Geometry: see drawing. Coordinates: mm, zero at the bounding-box minimum. A direction names the side the tool comes from. Give positions to 0.01 mm unless a question says otherwise; leave off trailing zeros. Write each loop counter-clockwise with the first axis right and the second up, starting at its lowest first coordinate (ties: lowest second). Pieces come first, ordered by that corner, then holes. Notation, with made-up numbers: (72, 10) -> (105, 10) arc R36 ccw to (105, 46) -> close; hole circle Ø1 at (50.25, 73.5). An arc over 180 degrees is marked (long way). Write item = value, one per line.
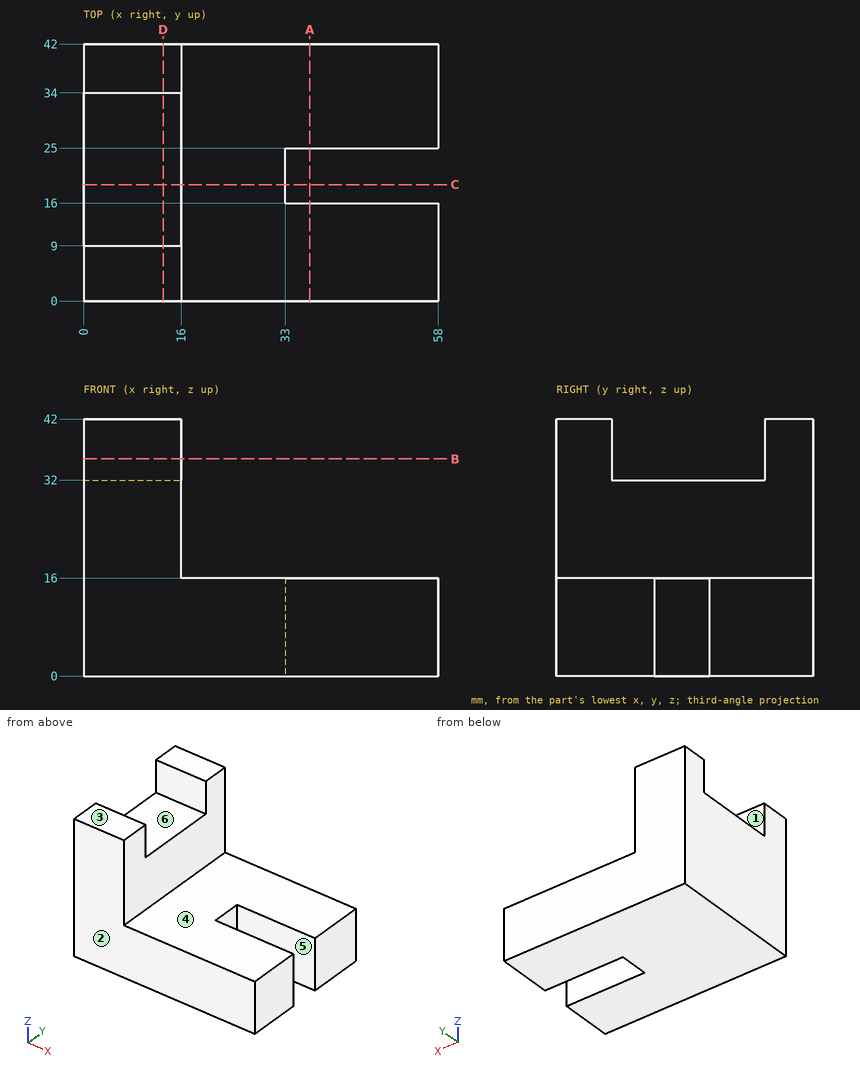
(1) Section query A-A (x = 37). Return loops of the section in (y, z), plus the area to 3 significant figures.
Values follow:
outline = (0, 0) -> (16, 0) -> (16, 16) -> (0, 16) -> close; (25, 0) -> (42, 0) -> (42, 16) -> (25, 16) -> close
area = 528 mm2
(2) Material intervals for line 1 (Y direction, x = 42.5, z = 10); line 2 (X direction, y = 24.5, z = 4); line 3 (X direction, y = 16, z = 29), sorted ascending.
Values follow:
line_1 = 0 to 16, 25 to 42
line_2 = 0 to 33
line_3 = 0 to 16
(3) Section query B-B (z = 35.5). Return loops of the section in (x, y).
Values follow:
outline = (0, 0) -> (16, 0) -> (16, 9) -> (0, 9) -> close; (0, 34) -> (16, 34) -> (16, 42) -> (0, 42) -> close
(4) Access query for the marked faces 4, 5 and 6. Directions: +Z, -Z, +X, -X, +Y, -Y. A direction counts if a zero-diameter tool reaches every point of the face in a straight line with its end or side. Return the directions, or none.
Values follow:
face_4 = +Z, +X, +Y, -Y
face_5 = +Z, -Z, +X
face_6 = +Z, +X, -X
(5) First-contact query: pin 1 (8 mm diameter, centred on x = 47, y = 18.5, fed in from +Z); pin 2 (4.5 mm diameter, centred on y = 19, z = 10, fed in from +X); pin 3 (5 mm diameter, centred on x = 4.5, y = 24, fed in from +Z). Flat tips, straight axial feed; report the tip coordinate or a pass-through.
Values follow:
pin_1 = 16
pin_2 = 33
pin_3 = 32
(6) Pull-direction query (Y, two-part tool) for the marked faces 1, 2 and 3; classes: pulls with the +Y half, pulls with the -Y half, needs draft (parallel to the pull), parting line crosses it, or undercut.
Values follow:
face_1 = undercut
face_2 = pulls with the -Y half
face_3 = needs draft
(7) Section query D-D (x = 13). Return loops of the section in (y, z).
Values follow:
outline = (0, 0) -> (42, 0) -> (42, 42) -> (34, 42) -> (34, 32) -> (9, 32) -> (9, 42) -> (0, 42) -> close
(8) Section query C-C (y = 19). Return loops of the section in (x, z).
Values follow:
outline = (0, 0) -> (33, 0) -> (33, 16) -> (16, 16) -> (16, 32) -> (0, 32) -> close
